```python
from build123d import *

# Parameters (mm, degrees)
SKETCH_1_R          = 4.5
EXTRUDE_1_DEPTH     = 4.5
CUT_EXTRUDE_1_DEPTH = 2
SKETCH_3_R          = 4
EXTRUDE_2_DEPTH     = 2.5
SKETCH_4_R          = 5
EXTRUDE_3_DEPTH     = 2
SKETCH_5_R          = 3
EXTRUDE_4_DEPTH     = 20
CHAMFER_1_SIZE      = 0.5
CHAMFER_2_SIZE      = 0.5
CHAMFER_3_SIZE      = 0.5
CHAMFER_4_SIZE      = 0.25


with BuildPart() as part:
    # ｽｹｯﾁ1 → ﾎﾞｽ - 押し出し1 (new body)
    with BuildSketch(Plane(origin=(0, 0, 0), x_dir=(1, 0, 0), z_dir=(0, 1, 0))):
        with Locations(Location((0, 0, 0), (0, 0, 270))):
            Circle(SKETCH_1_R)
    extrude(amount=EXTRUDE_1_DEPTH)

    # ｽｹｯﾁ2 → ｶｯﾄ - 押し出し1 (cut)
    with BuildSketch(Plane(origin=(0, 4.5, 0), x_dir=(1, 0, 0), z_dir=(0, 1, 0))):
        Polygon((2.886751346, 0), (1.443375673, 2.5), (-1.443375673, 2.5), (-2.886751346, 0), (-1.443375673, -2.5), (1.443375673, -2.5), align=None)
    extrude(amount=-CUT_EXTRUDE_1_DEPTH, mode=Mode.SUBTRACT)

    # ｽｹｯﾁ3 → ﾎﾞｽ - 押し出し2 (add)
    with BuildSketch(Plane.XZ):
        with Locations(Location((0, 0, 0), (0, 0, 90))):
            Circle(SKETCH_3_R)
    extrude(amount=EXTRUDE_2_DEPTH)

    # ｽｹｯﾁ4 → ﾎﾞｽ - 押し出し3 (add)
    with BuildSketch(Plane.XZ.offset(2.5)):
        with Locations(Location((0, 0, 0), (0, 0, 270))):
            Circle(SKETCH_4_R)
    extrude(amount=EXTRUDE_3_DEPTH)

    # ｽｹｯﾁ5 → ﾎﾞｽ - 押し出し4 (add)
    with BuildSketch(Plane.XZ.offset(4.5)):
        with Locations(Location((0, 0, 0), (0, 0, 270))):
            Circle(SKETCH_5_R)
    extrude(amount=EXTRUDE_4_DEPTH)

    # 面取り1
    chamfer_1_edges = [part.edges().sort_by_distance(p)[0] for p in [
        (0, 4.5, -4.5),
    ]]
    chamfer(chamfer_1_edges, length=CHAMFER_1_SIZE)

    # 面取り2
    chamfer_2_edges = [part.edges().sort_by_distance(p)[0] for p in [
        (0, 0, -4.5),
    ]]
    chamfer(chamfer_2_edges, length=CHAMFER_2_SIZE - 0.0001)  # a hair under: the kernel refuses the full size

    # 面取り3
    chamfer_3_edges = [part.edges().sort_by_distance(p)[0] for p in [
        (0, -2.5, 5),
        (0, -4.5, 5),
    ]]
    chamfer(chamfer_3_edges, length=CHAMFER_3_SIZE)

    # 面取り4
    chamfer_4_edges = [part.edges().sort_by_distance(p)[0] for p in [
        (2.165063509, 2.5, -1.25),
        (2.165063509, 4.5, 1.25),
        (2.165063509, 4.5, -1.25),
        (0, 4.5, -2.5),
        (-2.165063509, 4.5, -1.25),
        (-2.165063509, 4.5, 1.25),
        (0, 4.5, 2.5),
        (2.165063509, 2.5, 1.25),
        (0, 2.5, 2.5),
        (-2.165063509, 2.5, 1.25),
        (-2.165063509, 2.5, -1.25),
        (0, 2.5, -2.5),
    ]]
    chamfer(chamfer_4_edges, length=CHAMFER_4_SIZE)


solid = part.part
```
Verification items for the finished model (mm, model axes). A direction names the side the tool comes from. Coordinates: 2 decimals unless noted, no trailing zeros. Write each loop counter-clockwise with the first axis right and the second up, starting at its lowest first coordinate (ties: lowest second). Pieces come first, ordered by that corner, then holes. Notation, with made-up numbers: (17, 79) - (22, 79) arc R12 cw to (22, 94) - close; hole circle Ø11 at (-2, 13.5). An arc over 180 degrees is marked (long way). Write item = value, one per line.
Q1. Material ranges on L1, parallel to Y at x = -1.25, z = 3.25; L2, parallel to X at y = 3.25, z = -1; L3, parallel to Y at x = -1.25, z = 4, recorded low to high. Write a range as from..to.
Answer:
L1 = -4.5..4.5
L2 = -4.39..-2.31, 2.31..4.39
L3 = -4.5..-2.5, 0.19..4.31
Q2. Cross-section at B-B (y = -8.75). Enter the section's corners in (x, z).
Answer:
outline = circle Ø6 at (0, 0)
Q3. Mould release check, pull along Z, two halves, no side actions. Record for faces 1 (the face through (3.905, -1.232, -0.867)), 2 (the face through (2.26, 4.37, 1.33)), 3 (the face through (3, 4.5, 1)): released by +Z, released by -Z, zero draft, split by the parting line, or undercut.
Answer:
face_1 = split by the parting line
face_2 = undercut
face_3 = zero draft
Q4. Access from +Z, -Z, +X, -X, +Y, -Y to the whole of each face (thin tool, end or side, straight path). Record for faces 4 (the face through (-2.28, 4.37, 1.29)), 5 (the face through (0.9, -14.36, -2.86)), 6 (the face through (-3, -2.5, 3)).
Answer:
face_4 = +Y
face_5 = -Y
face_6 = none
Q5. Go/stop test with flat-tipped pins: pin 1 Ø1.2 at (x, y) = (-0.5, 3.5) entering from +Z; pin 2 Ø2 at (x, y) = (-2, -17) entering from -Z; pin 3 Ø3 at (y, z) = (-17.5, -3.5) entering from -X. Record where each tip stops, or that it passes through.
Answer:
pin_1 = 4.5
pin_2 = -2.83
pin_3 = -2.24
